from build123d import *

# Parameters (mm, degrees)
F0_W     = 120
F0_H     = 80
F1_DEPTH = 10
F2_R     = 5
F3_W     = 90
F3_H     = 60
F4_DEPTH = 5
F5_R     = 10
F7_D     = 7


with BuildPart() as f1:
    # F0 (on Top) → F1 (new body)
    with BuildSketch(Plane.XY):
        Rectangle(F0_W, F0_H)
    extrude(amount=F1_DEPTH)

    # F2
    f2_edges = [f1.edges().sort_by_distance(p)[0] for p in [
        (60, -40, 5),
        (60, 40, 5),
        (-60, -40, 5),
        (-60, 40, 5),
    ]]
    fillet(f2_edges, radius=F2_R)

    # F3 (on face) → F4 (cut)
    with BuildSketch(Plane.XY.offset(10)):
        Rectangle(F3_W, F3_H)
    extrude(amount=-F4_DEPTH, mode=Mode.SUBTRACT)

    # F5
    f5_edges = [f1.edges().sort_by_distance(p)[0] for p in [
        (-45, 30, 7.5),
        (45, 30, 7.5),
        (45, -30, 7.5),
        (-45, -30, 7.5),
    ]]
    fillet(f5_edges, radius=F5_R)

    # F7 (through all)
    with Locations(Plane.XY.offset(10)):
        with Locations((-55, -35), (-55, 35), (55, -35), (55, 35)):
            Hole(F7_D / 2)


solid = f1.part
Build history of the part. All positions in model axes, mm. A direction names the side the tool comes from. Give positions to 0.01 mm unless a question says otherwise; leave off trailing zeros. Order: outer loops, then holes, each group sorted by start corner. A loop starts at its lowest first (then second) coordinate and runs counter-clockwise, first axis right, second up. Notation, with made-up numbers: M -18.75,29.25 L 39.25,29.25 A21 ccw 39.25,62.25 Z; hole C 31,46 d4. An arc over 180 degrees is marked long. Put each result on its own line as item: value.
Item 1: Cut at C-C on x = -8.5. Write the cut outline in (y, z).
Results are:
outline: M -40,0 L 40,0 L 40,10 L 30,10 L 30,5 L -30,5 L -30,10 L -40,10 Z
Item 2: Pull direction Y, two halves, no side cores. Call faces 3 (the face through (-45, 0, 8)), 4 (the face through (60, 0, 5)), 5 (the face through (-59, -38, 5)): +Y half, -Y half, draft (parallel to the pull), parting line (faces both ways), or undercut.
Results are:
face 3: undercut
face 4: draft
face 5: -Y half
Item 3: Cut at A-A on z = 8.75. Write the cut outline in (x, y).
Results are:
outline: M -60,-35 A5 ccw -55,-40 L 55,-40 A5 ccw 60,-35 L 60,35 A5 ccw 55,40 L -55,40 A5 ccw -60,35 Z; hole C -55,-35 d7; hole C -55,35 d7; hole M -45,-20 A10 ccw -35,-30 L 35,-30 A10 ccw 45,-20 L 45,20 A10 ccw 35,30 L -35,30 A10 ccw -45,20 Z; hole C 55,-35 d7; hole C 55,35 d7
Item 4: Which spindle directions (+Z, -Z, +X, -X, +Y, -Y) get a long thin tool onto all of the face, cutting with end or side? Do faces 1 (the face through (59, 38, 5)), 2 (the face through (-41.99, -27.15, 7.46)). Say none if no direction does.
Results are:
face 1: +Z, -Z, +X, +Y
face 2: +Z
Item 5: Cut at B-B on y = 5.5. Write the cut outline in (x, z).
Results are:
outline: M -60,0 L 60,0 L 60,10 L 45,10 L 45,5 L -45,5 L -45,10 L -60,10 Z
Item 6: Wall check: probe 1 along Y at (x, z) = (55, 4.75); probe 2 along X at (y, z) = (7.5, 9); probe 3 along Z at (x, y) = (-21, 27). Give the ranges that are in metal, low to high.
Results are:
probe 1: -40 to -38.5, -31.5 to 31.5, 38.5 to 40
probe 2: -60 to -45, 45 to 60
probe 3: 0 to 5
Item 7: Drop a flat-ended pin along its axis: pin 1 Ø4 at (x, y) = (55, -35) entering from -Z. Give the stop position or say it passes through.
Results are:
pin 1: through
